from build123d import *

# Parameters (mm, degrees)
SKETCH1_W           = 25.4
SKETCH1_H           = 25.4
BOSS_EXTRUDE1_DEPTH = 2.54
BOSS_EXTRUDE2_DEPTH = 5.08
SKETCH3_R           = 5.053169443
CUT_EXTRUDE1_DEPTH  = 35.801810995


with BuildPart() as part:
    # Sketch1 → Boss-Extrude1 (new body)
    with BuildSketch(Plane(origin=(0, 0, 0), x_dir=(1, 0, 0), z_dir=(0, 1, 0))):
        Rectangle(SKETCH1_W, SKETCH1_H)
    extrude(amount=BOSS_EXTRUDE1_DEPTH)

    # Sketch2 → Boss-Extrude2 (add)
    with BuildSketch(Plane(origin=(12.7, 0, 0), x_dir=(0, 0, -1), z_dir=(1, 0, 0))):
        with BuildLine():
            Line((-12.7, 2.54), (-8.987628784, 16.394757994))
            ThreePointArc((-8.987628784, 16.394757994), (0, 20.11755573), (8.987628784, 16.394757994))
            Line((8.987628784, 16.394757994), (12.7, 2.54))
            Line((12.7, 2.54), (-12.7, 2.54))
        make_face()
    boss_extrude2 = extrude(amount=-BOSS_EXTRUDE2_DEPTH)

    # Mirror1: Boss-Extrude2 across plane
    add(boss_extrude2.mirror(Plane(origin=(0, 0, 0), x_dir=(0, 0, 1), z_dir=(1, 0, 0))))

    # Sketch3 → Cut-Extrude1 (cut, through all)
    with BuildSketch(Plane(origin=(12.7, 0, 0), x_dir=(0, 0, -1), z_dir=(1, 0, 0))):
        with Locations((0, 10.16)):
            Circle(SKETCH3_R)
    extrude(amount=-CUT_EXTRUDE1_DEPTH, mode=Mode.SUBTRACT)


solid = part.part
For this review, take the finished solid that the model builds, in its own axes (mm). A direction names the side the tool comes from. Give positions to 0.01 mm unless a question says otherwise; leave off trailing zeros. Order: outer loops, then holes, each group sorted by start corner. A loop starts at its lowest first (then second) coordinate and runs counter-clockwise, first axis right, second up. Notation, with made-up numbers: (-14, 2.25) - (14, 2.25) arc R29 cw to (14, 38.25) - close; hole circle Ø1 at (23.25, 45.5). An arc over 180 degrees is marked (long way). Answer as a JSON object with one key per item and string values. Group by question number.
Item 1: Machinability: for faces 4 (the flat face through (-10.2, 9.56, -10.82)), 5 (the flat face through (7.62, 15.4, -0.2)), which of the approach directions +Z, -Z, +X, -X, +Y, -Y give a long, thin tool a straight path to every point of the face, cutting with its end or side? Answer none if there is none.
Item 2: Take a section at A-A on x = 11. Give the boundary of the cut face in (y, z).
Item 3: Clearance check with flat-ended pins moving along their axes: pin 1 Ø3 at (x, y) = (7.5, 13.5) entering from +Z; pin 2 Ø5 at (x, y) = (8, 13) entering from +Z; pin 3 Ø5 at (x, y) = (-10, 11.5) entering from +Z. State where each tip first meets the part, or that it passes through.
Item 4: Take a section at D-D on z = 6. Give the boundary of the cut face in (x, y), and give its area (3 significant figures).
Item 5: Take a section at C-C on y = 7. Give the boundary of the cut face in (x, z), and give its area (3 significant figures).
Item 6: Wall thickness on line 1 along Y through (x, z) = (-8.85, 0); line 2 along X through (y, z) = (15.25, 7); line 3 along Y through (x, z) = (5.75, 10.25): over which ranges is each line inside the solid? List them lowest first.
Item 7: Draft analysis for pull direction X (two halves, no side actions). For faces 1 (the flat face through (-12.7, 5.7, -3)), 2 (the flat face through (-10.2, 9.37, 10.87)), 3 (the flat face through (-7.62, 15.4, -0.2)), state which applies: pulls with the +X half, pulls with the -X half, needs draft (parallel to the pull), parting line crosses it, or undercut.
Item 8: Take a section at B-B on z = 0. Give the boundary of the cut face in (x, y).
Reported:
{
 "1": {"face 4": "-Z, +X, -X, +Y", "face 5": "+Z, -Z, +Y"},
 "2": {"outline": "(0, -12.7) - (2.54, -12.7) - (16.39, -8.99) arc R12.71 ccw to (16.39, 8.99) - (2.54, 12.7) - (0, 12.7) - close; hole circle Ø10.11 at (10.16, 0)"},
 "3": {"pin 1": "z = 10.16", "pin 2": "z = 10.57", "pin 3": "z = 10.97"},
 "4": {"outline": "(-12.7, 0) - (12.7, 0) - (12.7, 18.61) - (7.62, 18.61) - (7.62, 2.54) - (-7.62, 2.54) - (-7.62, 18.61) - (-12.7, 18.61) - close", "area": "228 mm^2"},
 "5": {"outline": "(-12.7, -11.5) - (-7.62, -11.5) - (-7.62, -3.94) - (-12.7, -3.94) - close; (-12.7, 3.94) - (-7.62, 3.94) - (-7.62, 11.5) - (-12.7, 11.5) - close; (7.62, -11.5) - (12.7, -11.5) - (12.7, -3.94) - (7.62, -3.94) - close; (7.62, 3.94) - (12.7, 3.94) - (12.7, 11.5) - (7.62, 11.5) - close", "area": "154 mm^2"},
 "6": {"line 1": "0 to 5.11, 15.21 to 20.12", "line 2": "-12.7 to -7.62, 7.62 to 12.7", "line 3": "0 to 2.54"},
 "7": {"face 1": "pulls with the -X half", "face 2": "needs draft", "face 3": "undercut"},
 "8": {"outline": "(-12.7, 0) - (12.7, 0) - (12.7, 5.11) - (7.62, 5.11) - (7.62, 2.54) - (-7.62, 2.54) - (-7.62, 5.11) - (-12.7, 5.11) - close; (-12.7, 15.21) - (-7.62, 15.21) - (-7.62, 20.12) - (-12.7, 20.12) - close; (7.62, 15.21) - (12.7, 15.21) - (12.7, 20.12) - (7.62, 20.12) - close"}
}
